from build123d import *

# Parameters (mm, degrees)
F1_DEPTH  = 26
F2_W      = 46.52
F2_H      = 17.5
F3_DEPTH  = 53.901
F5_D      = 9
F5_DEPTH  = 12
F5_TIP    = 2.7038727856
F7_D      = 3.3
F7_DEPTH  = 30
F7_TIP    = 0.9914200214
F9_D      = 5
F9_DEPTH  = 12.5
F9_TIP    = 1.5021515476
F11_D     = 4.6
F11_DEPTH = 12.5
F11_TIP   = 1.3819794238
F10_R     = 2.3
F12_DEPTH = 13
F14_DEPTH = 26.001
F15_R     = 2


with BuildPart() as f1:
    # F0 (on Front) → F1 (new body)
    with BuildSketch(Plane.XZ):
        with BuildLine():
            Line((23.3, 53.9), (-29.4678404338, 53.9))
            ThreePointArc((-29.4678404338, 53.9), (-30.7588348825, 53.4275252317), (-31.4398670282, 52.2333333333))
            ThreePointArc((-31.4398670282, 52.2333333333), (-34.2289321881, 46.8289321881), (-39.6333333333, 44.0398670282))
            ThreePointArc((-39.6333333333, 44.0398670282), (-40.8275252317, 43.3588348825), (-41.3, 42.0678404338))
            Line((-41.3, 42.0678404338), (-41.3, 11.8321595662))
            ThreePointArc((-41.3, 11.8321595662), (-40.8275252317, 10.5411651175), (-39.6333333333, 9.8601329718))
            ThreePointArc((-39.6333333333, 9.8601329718), (-34.2289321881, 7.0710678119), (-31.4398670282, 1.6666666667))
            ThreePointArc((-31.4398670282, 1.6666666667), (-30.7588348825, 0.4724747683), (-29.4678404338, 0))
            Line((-29.4678404338, 0), (39.3, 0))
            ThreePointArc((39.3, 0), (40.7142135624, 0.5857864376), (41.3, 2))
            Line((41.3, 2), (41.3, 29.08))
            ThreePointArc((41.3, 29.08), (40.7142135624, 30.4942135624), (39.3, 31.08))
            Line((39.3, 31.08), (35.3, 31.08))
            ThreePointArc((35.3, 31.08), (28.2289321881, 34.0089321881), (25.3, 41.08))
            Line((25.3, 41.08), (25.3, 51.9))
            ThreePointArc((25.3, 51.9), (24.7142135624, 53.3142135624), (23.3, 53.9))
        make_face()
    extrude(amount=-F1_DEPTH)

    # F2 (on face) → F3 (cut, through all)
    with BuildSketch(Plane.XY.offset(53.9)):
        with Locations((-7.46, 13)):
            Rectangle(F2_W, F2_H)
    extrude(amount=-F3_DEPTH, mode=Mode.SUBTRACT)

    # F5
    with Locations(Plane.XZ):
        with Locations((-6.8, 26.9)):
            Hole(F5_D / 2, depth=F5_DEPTH)
            with Locations((0, 0, -(F5_DEPTH + F5_TIP / 2))):  # 118° drill point
                Cone(0, F5_D / 2, F5_TIP, mode=Mode.SUBTRACT)

    # F7
    with Locations(Plane.YZ.offset(41.3)):
        with Locations((13, 18.95), (13, 6.65)):
            Hole(F7_D / 2, depth=F7_DEPTH)
            with Locations((0, 0, -(F7_DEPTH + F7_TIP / 2))):  # 118° drill point
                Cone(0, F7_D / 2, F7_TIP, mode=Mode.SUBTRACT)

    # F9
    with Locations(Plane(origin=(0, 0, 0), x_dir=(1, 0, 0), z_dir=(0, 0, -1))):
        with Locations((36, -13), (21, -13)):
            Hole(F9_D / 2, depth=F9_DEPTH)
            with Locations((0, 0, -(F9_DEPTH + F9_TIP / 2))):  # 118° drill point
                Cone(0, F9_D / 2, F9_TIP, mode=Mode.SUBTRACT)

    # F11
    with Locations(Plane.XZ):
        with Locations((-9.6, 48.9), (-4.9, 5)):
            Hole(F11_D / 2, depth=F11_DEPTH)
            with Locations((0, 0, -(F11_DEPTH + F11_TIP / 2))):  # 118° drill point
                Cone(0, F11_D / 2, F11_TIP, mode=Mode.SUBTRACT)

    # F10 (on face) → F12 (join)
    with BuildSketch(Plane.XZ):
        with Locations((-9.6, 48.9)):
            Circle(F10_R)
        with Locations((-4.9, 5)):
            Circle(F10_R)
    extrude(amount=-F12_DEPTH)

    # F13 (on face) → F14 (cut, through all)
    with BuildSketch(Plane.XZ):
        with BuildLine():
            Line((-10.0679491924, 35.9), (-16.9961524227, 47.9))
            ThreePointArc((-16.9961524227, 47.9), (-18.7282032303, 48.9), (-20.4602540378, 47.9))
            Line((-20.4602540378, 47.9), (-27.3884572681, 35.9))
            ThreePointArc((-27.3884572681, 35.9), (-27.3884572681, 33.9), (-25.6564064606, 32.9))
            Line((-25.6564064606, 32.9), (-11.8, 32.9))
            ThreePointArc((-11.8, 32.9), (-10.0679491924, 33.9), (-10.0679491924, 35.9))
        make_face()
        with BuildLine():
            Line((12.0564064606, 48.9), (-1.8, 48.9))
            ThreePointArc((-1.8, 48.9), (-3.5320508076, 47.9), (-3.5320508076, 45.9))
            Line((-3.5320508076, 45.9), (3.3961524227, 33.9))
            ThreePointArc((3.3961524227, 33.9), (5.1282032303, 32.9), (6.8602540378, 33.9))
            Line((6.8602540378, 33.9), (13.7884572681, 45.9))
            ThreePointArc((13.7884572681, 45.9), (13.7884572681, 47.9), (12.0564064606, 48.9))
        make_face()
        with BuildLine():
            Line((-20.4602540378, 20), (-27.3884572681, 8))
            ThreePointArc((-27.3884572681, 8), (-27.3884572681, 6), (-25.6564064606, 5))
            Line((-25.6564064606, 5), (-11.8, 5))
            ThreePointArc((-11.8, 5), (-10.0679491924, 6), (-10.0679491924, 8))
            Line((-10.0679491924, 8), (-16.9961524227, 20))
            ThreePointArc((-16.9961524227, 20), (-18.7282032303, 21), (-20.4602540378, 20))
        make_face()
        with BuildLine():
            ThreePointArc((-1.8, 21), (-3.5320508076, 20), (-3.5320508076, 18))
            Line((-3.5320508076, 18), (3.3961524227, 6))
            ThreePointArc((3.3961524227, 6), (5.1282032303, 5), (6.8602540378, 6))
            Line((6.8602540378, 6), (13.7884572681, 18))
            ThreePointArc((13.7884572681, 18), (13.7884572681, 20), (12.0564064606, 21))
            Line((12.0564064606, 21), (-1.8, 21))
        make_face()
    extrude(amount=-F14_DEPTH, mode=Mode.SUBTRACT)

    # F15
    f15_edges = [f1.edges().sort_by_distance(p)[0] for p in [
        (-41.3, 13, 42.06784),
        (-41.3, 13, 11.83216),
        (-41.3, 0, 26.95),
        (-41.3, 26, 26.95),
    ]]
    fillet(f15_edges, radius=F15_R)


solid = f1.part
The listing builds one solid part. Answer for the finished solid, in the listing's coordinates (mm). A direction names the side the tool comes from. Give positions to 0.01 mm unless a question says otherwise; leave off trailing zeros. Order: outer loops, then holes, each group sorted by start corner. A loop starts at its lowest first (then second) coordinate and runs counter-clockwise, first axis right, second up. Notation, with made-up numbers: (79.5, -33) - (88.5, -33) arc R15 ccw to (88.5, -20) - close; hole circle Ø9 at (17, 64.5). An arc over 180 degrees is marked (long way). One line per item, written item: value. Start each with the question number.
1) A cutting plane is placed at D-D on z = 26.9. Give the vertices of the cut face in (x, y), then the cut area to 3 significant figures.
2) A tool of negligible diameter and unlimited length cuts with its end or side. For faces 1 (the face through (-8, 21.75, 27)), 2 (the face through (-18.7, 23.8, 21)), 3 (the face through (24.7, 0.57, 46.57)), 4 (the face through (37.27, 25.43, 30.48)), from which of +Z, -Z, +X, -X, +Y, -Y can it reach the whole face along a straight path? Write none if from no direction.
3) A cutting plane is placed at A-A on y = 19. Give the vertices of the cut face in (x, z).
4) A cutting plane is placed at B-B on z = 18.95. State how many separate pieces and enclosed holes the cut face has, then the cut area to 3 significant figures.
5) The mould has two halves that part along X. Classify faces 5 (the face through (37.27, 0.57, 30.48)), 6 (the face through (40.7, 25.43, 15.73)), 7 (the face through (-3.517, 2.095, 20.025)): released by +X, released by -X, zero draft, split by the parting line, or undercut.
6) Find the intervals of material crossed by L1, parallel to Y at x = 15, z = 42.5; L2, parallel to Z at x = 32.5, y = 13; L3, parallel to Z at x = -6.8, y = 1.9, in increasing order.
7) A cutting plane is placed at C-C on x = -4.9. Give the vertices of the cut face in (y, z), then the cut area to 3 significant figures.
8) Given pin 1 Ø8 at (y, z) = (10, 41) entering from +X; pin 2 Ø1 at (y, z) = (6.5, 48) entering from +X; pin 3 Ø2 at (y, z) = (13, 6.65) entering from +X, each flat-ended and moving along its own axis, determine where each tip first touches the part or whether it passes through.
Answer sheet:
1. outline: (-41.3, 2) arc R2 ccw to (-39.3, 0) - (-11.3, 0) - (-11.3, 4.25) - (-30.72, 4.25) - (-30.72, 21.75) - (15.8, 21.75) - (15.8, 4.25) - (-2.3, 4.25) - (-2.3, 0) - (39.3, 0) arc R2 ccw to (41.3, 2) - (41.3, 24) arc R2 ccw to (39.3, 26) - (-39.3, 26) arc R2 ccw to (-41.3, 24) - close
1. area: 1,290 mm2
2. face 1: +Z, -Z
2. face 2: +Y, -Y
2. face 3: +Z, +X, -Y
2. face 4: +Z, +X, +Y
3. outline: (-41.3, 11.83) arc R2 ccw to (-39.63, 9.86) arc R10 cw to (-31.44, 1.67) arc R2 ccw to (-30.72, 0.44) - (-30.72, 53.46) arc R2 ccw to (-31.44, 52.23) arc R10 cw to (-39.63, 44.04) arc R2 ccw to (-41.3, 42.07) - close; (15.8, 0) - (39.3, 0) arc R2 ccw to (41.3, 2) - (41.3, 29.08) arc R2 ccw to (39.3, 31.08) - (35.3, 31.08) arc R10 cw to (25.3, 41.08) - (25.3, 51.9) arc R2 ccw to (23.3, 53.9) - (15.8, 53.9) - close
4. separate pieces: 5
4. enclosed holes: 0
4. area: 1,050 mm2
5. face 5: zero draft
5. face 6: released by +X
5. face 7: undercut
6. L1: y = 0 to 4.25, 21.75 to 26
6. L2: z = 0 to 5, 8.3 to 17.3, 20.6 to 31.48
6. L3: z = 0 to 22.4, 31.4 to 53.9
7. outline: (0, 2) arc R2 ccw to (2, 0) - (4.25, 0) - (4.25, 2.7) - (13, 2.7) - (13, 7.3) - (4.25, 7.3) - (4.25, 22.82) - (0, 22.82) - close; (0, 30.98) - (4.25, 30.98) - (4.25, 53.9) - (2, 53.9) arc R2 ccw to (0, 51.9) - close; (21.75, 0) - (24, 0) arc R2 ccw to (26, 2) - (26, 51.9) arc R2 ccw to (24, 53.9) - (21.75, 53.9) - close
7. area: 460 mm2
8. pin 1: stops at x = 26.17
8. pin 2: stops at x = 25.3
8. pin 3: stops at x = -2.69
